```python
from build123d import *

# Parameters (mm, degrees)
SKETCH2_R           = 4
CUT_EXTRUDE1_DEPTH  = 6.5
SKETCH3_W           = 14.803302618
SKETCH3_H           = 22
BOSS_EXTRUDE1_DEPTH = 11.5
BOSS_EXTRUDE2_DEPTH = 2


with BuildPart() as part:
    # Sketch1 → Revolve1 (revolve)
    with BuildSketch(Plane.XY, mode=Mode.PRIVATE) as revolve1_sk:
        Polygon((0, 20.572271817), (-8, 20.572271817), (-8, 16.872271817), (-6, 16.872271817), (-6, 10.872271817), (-8, 10.872271817), (-8, 7.872271817), (-5.267364971, 7.872271817), (-5.267364971, 6.372271817), (-8, 6.372271817), (-8, 5.372271817), (-5.001966623, 5.372271817), (-5.001966623, 3.872271817), (-11.15, 3.872271817), (-11.15, 2.872271817), (-5.001966623, 2.872271817), (-5.001966623, 1.372271817), (-11.15, 1.372271817), (-11.15, 0.372271817), (-5.001966623, 0.372271817), (-5.001966623, -1.127728183), (-11.15, -1.127728183), (-11.15, -2.127728183), (-5.001966623, -2.127728183), (-5.001966623, -3.627728183), (-11.15, -3.627728183), (-11.15, -4.627728183), (-5.001966623, -4.627728183), (-5.001966623, -6.127728183), (-11.15, -6.127728183), (-11.15, -7.127728183), (-5.001966623, -7.127728183), (-5.001966623, -8.627728183), (-11.15, -8.627728183), (-11.15, -9.627728183), (-5.001966623, -9.627728183), (-5.001966623, -11.127728183), (-11.15, -11.127728183), (-11.15, -12.127728183), (-5.001966623, -12.127728183), (-5.001966623, -13.627728183), (-11.15, -13.627728183), (-11.15, -14.627728183), (-5.001966623, -14.627728183), (-5.001966623, -16.127728183), (-11.15, -16.127728183), (-11.15, -17.127728183), (-5.001966623, -17.127728183), (-5.001966623, -18.627728183), (-11.15, -18.627728183), (-11.15, -19.627728183), (-5.001966623, -19.627728183), (-5.001966623, -21.127728183), (-11.15, -21.127728183), (-11.15, -22.127728183), (-5.001966623, -22.127728183), (-3, -22.127728183), (-3, -39.714128425), (-0.738340975, -41.627728183), (0, -41.627728183), (0, -33.805569091), align=None)
    revolve(revolve1_sk.sketch.rotate(Axis((0, 0, 0), (0, 1, 0)), 180), axis=Axis((0, 0, 0), (0, 1, 0)))

    # Sketch2 → Cut-Extrude1 (cut)
    with BuildSketch(Plane(origin=(0, 20.572271817, 0), x_dir=(1, 0, 0), z_dir=(0, 1, 0))):
        with Locations(Location((0, 0, 0), (0, 0, 180))):
            Circle(SKETCH2_R)
    extrude(amount=-CUT_EXTRUDE1_DEPTH, mode=Mode.SUBTRACT)

    # Sketch3 → Boss-Extrude1 (add)
    with BuildSketch(Plane(origin=(0, -24.127728183, 0), x_dir=(-1, 0, 0), z_dir=(0, -1, 0))):
        with Locations((0, -4.5)):
            Rectangle(SKETCH3_W, SKETCH3_H)
    extrude(amount=BOSS_EXTRUDE1_DEPTH)

    # Sketch4 → Boss-Extrude2 (add)
    with BuildSketch(Plane(origin=(0, -35.627728183, 0), x_dir=(-1, 0, 0), z_dir=(0, -1, 0))):
        Polygon((4.730605377, 0), (2.365302689, 4.096824432), (-2.365302689, 4.096824432), (-4.730605377, 0), (-2.365302689, -4.096824432), (2.365302689, -4.096824432), align=None)
    extrude(amount=BOSS_EXTRUDE2_DEPTH)


solid = part.part
```
For this review, take the finished solid that the model builds, in its own axes (mm). A direction names the side the tool comes from. Coordinates: 2 decimals unless noted, no trailing zeros. Order: outer loops, then holes, each group sorted by start corner. A loop starts at its lowest first (then second) coordinate and runs counter-clockwise, first axis right, second up. Notation, with made-up numbers: (-22, 24.25) -> (6, 24.25) arc R8 cw to (6, 29.25) -> close; hole circle Ø7 at (-10.5, -22.5). An arc over 180 degrees is marked (long way). Use CSV: the item, a comma, the result in double quotes. Start each with the question number.
Item 1: We need section A-A, the plane x = 8.75. Give the number of separate pieces and of enclosed holes in the cut face, then the cut area to 3 significant figures.
Item 2: We need section B-B, the plane y = 2. Give the boundary of the cut face in (x, z), then the cut area to 3 significant figures.
Item 3: Draft analysis for pull direction Y (two halves, no side actions). For faces 1 (the face through (2, 10.872, -6)), 2 (the face through (0.1, -35.628, 4.3)), 3 (the face through (-1.73, 9.35, 7.81)), state which applies: pulls with the +Y half, pulls with the -Y half, needs draft (parallel to the pull), parting line crosses it, or undercut.
Item 4: Insertion check: pin 1 (12 mm diameter, centred on y = 13, z = -0.5, fed in from +X); pin 2 (6 mm diameter, centred on x = -3.5, y = -28, fed in from -Z); pin 3 (2 mm diameter, centred on y = -31.5, z = 9.5, fed in from +X). Each pin has a flat end and moves straight along its axis. Give the tip position at first contact, or say it passes through.
Item 5: For faces 4 (the face through (0, -37, -4.097)), 5 (the face through (-5, 0, 0)), 6 (the face through (-1.73, 5.87, 7.81)), list the 3-axis set-ups (+Z, -Z, +X, -X, +Y, -Y) from which the entire face can be reached by the end or side of a thin tool; tool diameter is ignored.
Item 6: Wall thickness on probe 1 along Z at (x, y) = (0, 17.75); probe 2 along Z at (x, y) = (0, 16.5); probe 3 along Z at (x, y) = (6, -26.5): over which ranges is each line inside the solid? List them lowest first.
Derived:
1,separate pieces,"11"
1,enclosed holes,"0"
1,area,"152 mm^2"
2,outline,"circle Ø10 at (0, 0)"
2,area,"78.6 mm^2"
3,face 1,"undercut"
3,face 2,"pulls with the -Y half"
3,face 3,"needs draft"
4,pin 1,"stops at x = 8"
4,pin 2,"stops at z = -6.5"
4,pin 3,"stops at x = 7.4"
5,face 4,"-Z, +X, -X, -Y"
5,face 5,"none"
5,face 6,"+Y"
6,probe 1,"z = -8 to -4, 4 to 8"
6,probe 2,"z = -6 to -4, 4 to 6"
6,probe 3,"z = -6.5 to 15.5"
